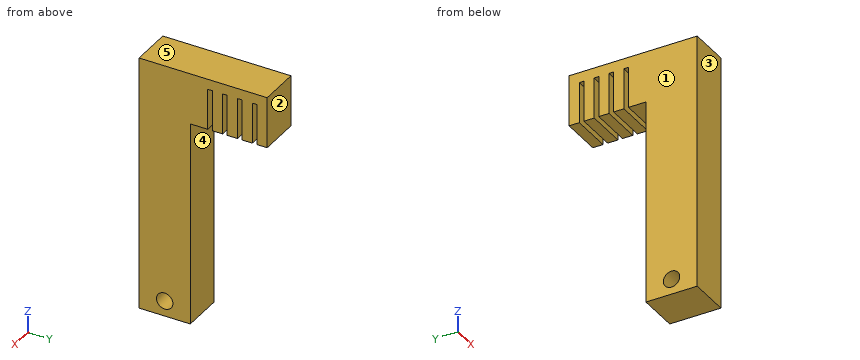
```python
from build123d import *

# Parameters (mm, degrees)
F0_W     = 8
F0_H     = 25
F1_DEPTH = 10
F2_W     = 8
F2_H     = 0.9
F3_DEPTH = 8
F4_W     = 8
F4_H     = 10
F5_DEPTH = 40
F6_R     = 1.6
F7_DEPTH = 8.001


with BuildPart() as f1:
    # F0 (on Top) → F1 (new body)
    with BuildSketch(Plane.XY):
        Rectangle(F0_W, F0_H)
    extrude(amount=F1_DEPTH)

    # F2 (on face) → F3 (cut)
    with BuildSketch(Plane(origin=(0, 0, 0), x_dir=(1, 0, 0), z_dir=(0, 0, -1))):
        with Locations((0, -10.05)):
            Rectangle(F2_W, F2_H)
        with Locations((0, -7.15)):
            Rectangle(F2_W, F2_H)
        with Locations((0, -4.25)):
            Rectangle(F2_W, F2_H)
        with Locations((0, -1.35)):
            Rectangle(F2_W, F2_H)
    extrude(amount=-F3_DEPTH, mode=Mode.SUBTRACT)

    # F4 (on face) → F5 (join)
    with BuildSketch(Plane(origin=(0, 0, 0), x_dir=(1, 0, 0), z_dir=(0, 0, -1))):
        with Locations((0, 7.5)):
            Rectangle(F4_W, F4_H)
    extrude(amount=F5_DEPTH)

    # F6 (on face) → F7 (cut, through all)
    with BuildSketch(Plane(origin=(-4, 0, 0), x_dir=(0, -1, 0), z_dir=(-1, 0, 0))):
        with Locations((7.5, -37)):
            Circle(F6_R)
    extrude(amount=-F7_DEPTH, mode=Mode.SUBTRACT)


solid = f1.part
```
Model file for the job. Use its own axes, mm. Face numbers are marked on the shaded views. A direction names the side the tool comes from. Coordinates: 2 decimals unless noted, no trailing zeros. Order: outer loops, then holes, each group sorted by start corner. A loop starts at its lowest first (then second) coordinate and runs counter-clockwise, first axis right, second up. Notation, with made-up numbers: (21.5, 69) -> (44.5, 69) arc R36 ccw to (44.5, 103) -> close; hole circle Ø7 at (75.5, -27). An arc over 180 degrees is marked (long way). Answer as a JSON object with one key per item and string values. Group by question number.
1) Drill centre lines: L1, parallel to Y at x = 1, z = 1.5; L2, parallel to Z at x = 1.75, y = -7.5; L3, parallel to Z at x = -0.75, y = -1.75. Where is each one in solid material? Low to high.
2) Cut at D-D, the plane z = -15. Write the cut outline in (x, y), then the cut area to 3 significant figures.
3) Cut at A-A, the plane z = -37. Write the cut outline in (x, y).
4) Pull direction Y, two halves, no side cores. Call the marked faces 1, 2 and 3: +Y half, -Y half, draft (parallel to the pull), parting line (faces both ways), or undercut.
5) Cut at B-B, the plane y = -7.5. Write the cut outline in (x, z), then the cut area to 3 significant figures.
6) Flat gauge pins, fed straight in: pin 1 (1 mm diameter, centred on x = 0.5, y = 9, fed in from -Z); pin 2 (10 mm diameter, centred on y = 2, z = -12.5, fed in from -X); pin 3 (4 mm diameter, centred on x = -1.5, z = -19, fed in from +Y). Where does each tip first touch, or does it go through?
7) Cut at C-C, the plane x = 1.75. Write the cut outline in (y, z), then the cut area to 3 significant figures.
8) Which spindle directions (+Z, -Z, +X, -X, +Y, -Y) get a long thin tool onto all of the face, cutting with end or side? Do the marked faces 4 and 5. Say none if no direction does.
Check values:
{
 "1": {"L1": "y = -12.5 to 0.9, 1.8 to 3.8, 4.7 to 6.7, 7.6 to 9.6, 10.5 to 12.5", "L2": "z = -40 to -38.6, -35.4 to 10", "L3": "z = 0 to 10"},
 "2": {"outline": "(-4, -12.5) -> (4, -12.5) -> (4, -2.5) -> (-4, -2.5) -> close", "area": "80.0 mm²"},
 "3": {"outline": "(-4, -12.5) -> (4, -12.5) -> (4, -9.1) -> (-4, -9.1) -> close; (-4, -5.9) -> (4, -5.9) -> (4, -2.5) -> (-4, -2.5) -> close"},
 "4": {"face 1": "draft", "face 2": "+Y half", "face 3": "-Y half"},
 "5": {"outline": "(-4, -40) -> (4, -40) -> (4, -38.6) -> (-4, -38.6) -> close; (-4, -35.4) -> (4, -35.4) -> (4, 10) -> (-4, 10) -> close", "area": "374 mm²"},
 "6": {"pin 1": "stops at z = 0", "pin 2": "stops at x = -4", "pin 3": "stops at y = -2.5"},
 "7": {"outline": "(-12.5, -40) -> (-2.5, -40) -> (-2.5, 0) -> (0.9, 0) -> (0.9, 8) -> (1.8, 8) -> (1.8, 0) -> (3.8, 0) -> (3.8, 8) -> (4.7, 8) -> (4.7, 0) -> (6.7, 0) -> (6.7, 8) -> (7.6, 8) -> (7.6, 0) -> (9.6, 0) -> (9.6, 8) -> (10.5, 8) -> (10.5, 0) -> (12.5, 0) -> (12.5, 10) -> (-12.5, 10) -> close; hole circle Ø3.2 at (-7.5, -37)", "area": "613 mm²"},
 "8": {"face 4": "-Z, +X, -X, +Y", "face 5": "+Z, +X, -X, +Y, -Y"}
}
